Part model, mm, in its own coordinate system. Face numbers are marked on the shaded views. A direction names the side the tool comes from. Give positions to 0.01 mm unless a question says otherwise; leave off trailing zeros. Write each loop counter-clockwise with the first axis right and the second up, starting at its lowest first coordinate (ties: lowest second). Pieces come first, ordered by that corner, then holes. Notation, with made-up numbers: M 14.5,71 L 54.5,71 A20 ccw 54.5,83 Z; hole C 39.5,-25.75 d10. An arc over 180 degrees is marked long. Use a Markdown table: item, result.
```python
from build123d import *

# Parameters (mm, degrees)
F0_W     = 81.28
F0_H     = 81.28
F0_W_2   = 50.377
F0_H_2   = 54.727
F1_DEPTH = 9.525
F3_D     = 3.175
F4_D     = 1.6002


# Not quite as in the source:
# - a feature names something its author has since deleted; it is built from what else it names


with BuildPart() as f1:
    # F0 (on Front) → F1 (new body)
    with BuildSketch(Plane.XZ):
        Rectangle(F0_W, F0_H)
        Rectangle(F0_W_2, F0_H_2, mode=Mode.SUBTRACT)
    extrude(amount=F1_DEPTH)

    # F3 (through all)
    with Locations(Plane.XZ.offset(9.525)):
        with Locations((-33.6692971992, 35.1226272138), (33.6692971992, 35.1226272138), (-33.6692971992, -35.1226272138), (33.6692971992, -35.1226272138)):
            Hole(F3_D / 2)

    # F4 (through all)
    with Locations(Plane(origin=(0, 0, 0), x_dir=(1, 0, 0), z_dir=(0, 1, 0))):
        with Locations((25.1885, -27.3635), (-25.1885, -27.3635), (-25.1885, 27.3635), (25.1885, 27.3635)):
            Hole(F4_D / 2)


solid = f1.part
```
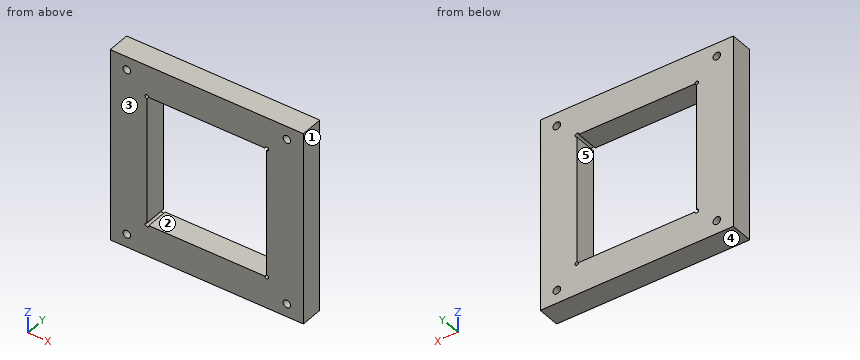
1. Cut at C-C, the plane y = -6.5. Give the cut face in (x, z) (1 decimal).
Findings below:
| item | result |
|---|---|
| outline | M -40.6,-40.6 L 40.6,-40.6 L 40.6,40.6 L -40.6,40.6 Z; hole C -33.7,-35.1 d3.2; hole C -33.7,35.1 d3.2; hole M -25.2,-26.6 A0.8 ccw long -24.4,-27.4 L 24.4,-27.4 A0.8 ccw long 25.2,-26.6 L 25.2,26.6 A0.8 ccw long 24.4,27.4 L -24.4,27.4 A0.8 ccw long -25.2,26.6 Z; hole C 33.7,-35.1 d3.2; hole C 33.7,35.1 d3.2 |
2. Two-plate mould, pull along X, no slides. Class the marked faces 1, 2 and 3: released by +X, released by -X, zero draft, split by the parting line, or undercut.
Findings below:
| item | result |
|---|---|
| face 1 | released by +X |
| face 2 | undercut |
| face 3 | zero draft |
3. Cut at B-B, the plane x = 10.5. Give the cut face in (y, z) (1 decimal), then the cut area to 3 significant figures.
Findings below:
| item | result |
|---|---|
| outline | M -9.5,-40.6 L 0,-40.6 L 0,-27.4 L -9.5,-27.4 Z; M -9.5,27.4 L 0,27.4 L 0,40.6 L -9.5,40.6 Z |
| area | 253 mm2 |
4. Tool access for the marked faces 4 and 5: list every direction of +Z, -Z, +X, -X, +Y, -Y with a clear straight run to the whole face (end or side of a thin tool).
Findings below:
| item | result |
|---|---|
| face 4 | -Z, +X, -X, +Y, -Y |
| face 5 | +Y, -Y |
5. Drill centre lines: L1, parallel to X at y = -1, z = -35; L2, parallel to Z at x = 7, y = -5.5; L3, parallel to X at y = -6.75, z = 12. Where is each one in solid material? Low to high.
Findings below:
| item | result |
|---|---|
| L1 | -40.64 to -35.25, -32.09 to 32.09, 35.25 to 40.64 |
| L2 | -40.64 to -27.36, 27.36 to 40.64 |
| L3 | -40.64 to -25.19, 25.19 to 40.64 |
6. Drop flat-ended pins along their axis: P1, Ø8, axis at x = 0.5, z = -24, coming from the +Y side; P2, Ø1.3, axis at x = 25.19, z = 27.36, coming from the -Y side. Give the stop position or say it passes through.
Findings below:
| item | result |
|---|---|
| P1 | y = 0 |
| P2 | through |
7. Cut at A-A, the plane z = 9.5. Give the cut face in (x, y) (1 decimal), then the cut area to 3 significant figures.
Findings below:
| item | result |
|---|---|
| outline | M -40.6,-9.5 L -25.2,-9.5 L -25.2,0 L -40.6,0 Z; M 25.2,-9.5 L 40.6,-9.5 L 40.6,0 L 25.2,0 Z |
| area | 294 mm2 |
